Design review of the part built by this model. Coordinates are the model's own, in mm. Face numbers are marked on the shaded views. Coordinates: 2 decimals unless noted, no trailing zeros. Write each loop counter-clockwise with the first axis right and the second up, starting at its lowest first coordinate (ties: lowest second). Pieces come first, ordered by that corner, then holes. Notation, with made-up numbers: M -29,-26 L 4,-26 A29 ccw 4,1 Z; hole C 32,-30 d6. An arc over 180 degrees is marked long. One line per question, with ' | ' between items.
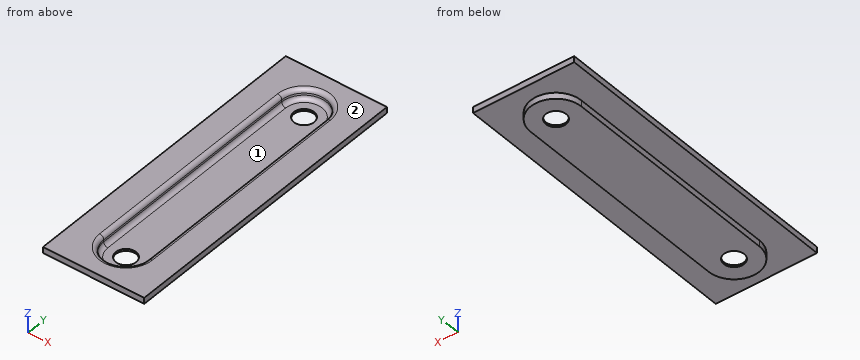
from build123d import *

# Parameters (mm, degrees)
F0_W     = 50
F0_H     = 150
F1_DEPTH = 3
F4_DEPTH = 6
F2_R     = 5
F5_DEPTH = 6.001
F6_DEPTH = 5
F7_R     = 2


with BuildPart() as f1:
    # F0 (on Top) → F1 (new body)
    with BuildSketch(Plane.XY):
        with Locations((25, 75)):
            Rectangle(F0_W, F0_H)
    extrude(amount=F1_DEPTH)

    # F3 (on face) → F4 (join)
    with BuildSketch(Plane.XY.offset(3)):
        with BuildLine():
            Line((37.5, 20), (37.5, 130))
            ThreePointArc((37.5, 130), (25, 142.5), (12.5, 130))
            Line((12.5, 130), (12.5, 20))
            ThreePointArc((12.5, 20), (25, 7.5), (37.5, 20))
        make_face()
        with BuildLine():
            ThreePointArc((36, 20), (25, 9), (14, 20))
            Line((14, 20), (14, 130))
            ThreePointArc((14, 130), (25, 141), (36, 130))
            Line((36, 130), (36, 20))
        make_face(mode=Mode.SUBTRACT)
        with BuildLine():
            Line((14, 130), (14, 20))
            ThreePointArc((14, 20), (25, 9), (36, 20))
            Line((36, 20), (36, 130))
            ThreePointArc((36, 130), (25, 141), (14, 130))
        make_face()
    extrude(amount=-F4_DEPTH)

    # F2 (on face) → F5 (cut, through all)
    with BuildSketch(Plane.XY.offset(3)):
        with Locations((25, 20)):
            Circle(F2_R)
        with Locations((25, 130)):
            Circle(F2_R)
    extrude(amount=-F5_DEPTH, mode=Mode.SUBTRACT)

    # F3 (on face) → F6 (cut)
    with BuildSketch(Plane.XY.offset(3)):
        with BuildLine():
            Line((14, 130), (14, 20))
            ThreePointArc((14, 20), (25, 9), (36, 20))
            Line((36, 20), (36, 130))
            ThreePointArc((36, 130), (25, 141), (14, 130))
        make_face()
    extrude(amount=-F6_DEPTH, mode=Mode.SUBTRACT)

    # F7
    f7_edges = [f1.edges().sort_by_distance(p)[0] for p in [
        (14, 75, 3),
        (14, 75, -2),
    ]]
    fillet(f7_edges, radius=F7_R)


solid = f1.part
1. Draft analysis for pull direction X (two halves, no side actions). For the marked faces 1 and 2, state which applies: pulls with the +X half, pulls with the -X half, needs draft (parallel to the pull), parting line crosses it, or undercut.
Answer sheet:
face 1: undercut | face 2: needs draft
2. To check wall thickness, follow line 1 along Y through (x, z) = (25, -2.3); line 2 along X through (y, z) = (86, 0.65); line 3 along Z through (x, y) = (40, 104.5). State the ranges of each line that lie inside material, in increasing order. Write a range as [from, to].
Answer sheet:
line 1: [7.5, 15], [25, 125], [135, 142.5] | line 2: [0, 14], [36, 50] | line 3: [0, 3]
3. Take a section at C-C (z = 2.05). Write out the cut boundary in (x, y), then the cut area to 3 significant figures.
Answer sheet:
outline: M 0,0 L 50,0 L 50,150 L 0,150 Z; hole M 13.7,20 A11.3 ccw 36.3,20 L 36.3,130 A11.3 ccw 13.7,130 Z | area: 4,610 mm^2
4. Take a section at A-A (x = 25). Write out the cut boundary in (y, z), then the cut area to 3 significant figures.
Answer sheet:
outline: M 0,0 L 7.5,0 L 7.5,-3 L 15,-3 L 15,-2 L 11,-2 A2 cw 9,0 L 9,1 A2 ccw 7,3 L 0,3 Z; M 25,-3 L 125,-3 L 125,-2 L 25,-2 Z; M 135,-3 L 142.5,-3 L 142.5,0 L 150,0 L 150,3 L 143,3 A2 ccw 141,1 L 141,0 A2 cw 139,-2 L 135,-2 Z | area: 175 mm^2
5. Take a section at B-B (y = 36). Write out the cut boundary in (x, z).
Answer sheet:
outline: M 0,0 L 12.5,0 L 12.5,-3 L 37.5,-3 L 37.5,0 L 50,0 L 50,3 L 38,3 A2 ccw 36,1 L 36,0 A2 cw 34,-2 L 16,-2 A2 cw 14,0 L 14,1 A2 ccw 12,3 L 0,3 Z
6. Insertion check: pin 1 Ø5 at (x, y) = (8, 100) entering from -Z; pin 2 Ø13 at (x, y) = (25, 20) entering from -Z; pin 3 Ø9 at (x, y) = (24.5, 68) entering from +Z; pin 4 Ø3 at (y, z) = (59.5, -2.5) entering from +X. Each pin has a flat end and moves straight along its axis. Give the tip position at first contact, or say it passes through.
Answer sheet:
pin 1: z = 0 | pin 2: z = -3 | pin 3: z = -2 | pin 4: x = 37.5
